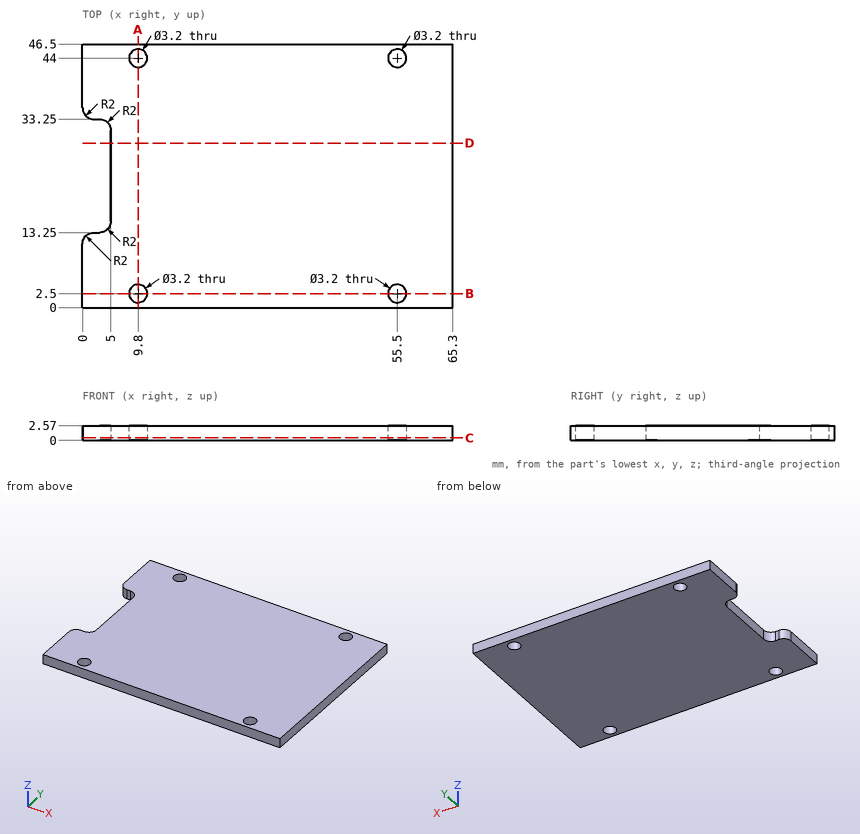
Drawing for the job (mm, zero at the part's lowest x, y, z). Give positions to 0.01 mm unless a question says otherwise; leave off trailing zeros. Order: outer loops, then holes, each group sorted by start corner. A loop starts at its lowest first (then second) coordinate and runs counter-clockwise, first axis right, second up. Notation, with made-up numbers: (77, -24) - (107, -24) arc R21 cw to (107, 2) - close; hole circle Ø2 at (-11, 58). An arc over 180 degrees is marked (long way). Use one line per item in the form item = value.
Item 1: Probe probe 1 along Y at (x, z) = (55.5, 1.1); probe 2 along Y at (x, z) = (3, 1); probe 3 along X at (y, z) = (35, 0.35). List the from-to ranges inside material, lowest first. Write a range as from..to.
Solution:
probe_1 = 0..0.9, 4.1..42.4, 45.6..46.5
probe_2 = 0..13.25, 33.25..46.5
probe_3 = 0.02..65.3
Item 2: Pin check, flat tips, straight feed: pin 1 Ø2 at (x, y) = (9, 41.5) entering from -Z; pin 2 Ø1.9 at (x, y) = (55.5, 44) entering from +Z. Stop position of each tip, or through.
Solution:
pin_1 = 0
pin_2 = through
Item 3: Slice it at B-B on y = 2.5. Give the cut face in (x, z).
Solution:
outline = (0, 0) - (8.2, 0) - (8.2, 2.57) - (0, 2.57) - close; (11.4, 0) - (53.9, 0) - (53.9, 2.57) - (11.4, 2.57) - close; (57.1, 0) - (65.3, 0) - (65.3, 2.57) - (57.1, 2.57) - close
Item 4: Slice it at C-C on z = 0.4. Give the cut face in (x, y), and give its area (3 significant figures).
Solution:
outline = (0, 0) - (65.3, 0) - (65.3, 46.5) - (0, 46.5) - (0, 35.25) arc R2 ccw to (2, 33.25) - (3, 33.25) arc R2 cw to (5, 31.25) - (5, 15.25) arc R2 cw to (3, 13.25) - (2, 13.25) arc R2 ccw to (0, 11.25) - close; hole circle Ø3.2 at (9.8, 2.5); hole circle Ø3.2 at (9.8, 44); hole circle Ø3.2 at (55.5, 2.5); hole circle Ø3.2 at (55.5, 44)
area = 2,900 mm2
Item 5: Slice it at A-A on x = 9.8. Give the cut face in (y, z).
Solution:
outline = (0, 0) - (0.9, 0) - (0.9, 2.57) - (0, 2.57) - close; (4.1, 0) - (42.4, 0) - (42.4, 2.57) - (4.1, 2.57) - close; (45.6, 0) - (46.5, 0) - (46.5, 2.57) - (45.6, 2.57) - close
Item 6: Slice it at D-D on y = 29. Give the cut face in (x, z).
Solution:
outline = (5, 0) - (65.3, 0) - (65.3, 2.57) - (5, 2.57) - close
